Can you work these out from the model? Positions are in its coordinate system, mm. Round coordinates to 2 decimals unless told otherwise and drop trailing zeros. Order: outer loops, then holes, each group sorted by start corner. A loop starts at its lowest first (then second) coordinate and runs counter-clockwise, first axis right, second up. Notation, with made-up numbers: M 63,4.25 L 95,4.25 A23 cw 95,28.25 Z; hole C -4.5,44 d3. An arc over 180 degrees is marked long. Answer as CSV lines item,"result". Start each with the question number.
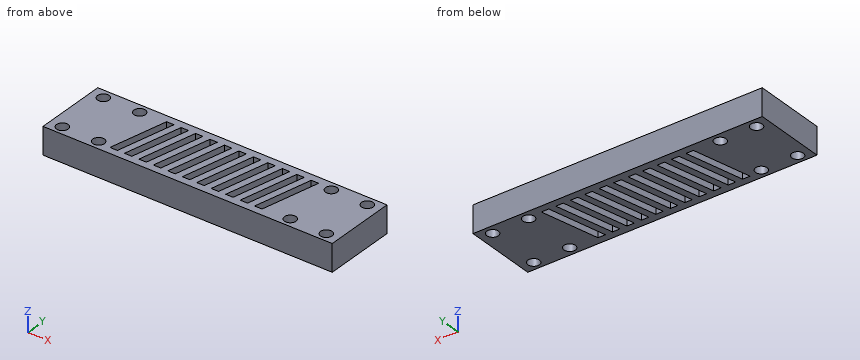
from build123d import *

# Parameters (mm, degrees)
SKETCH1_W           = 80
SKETCH1_H           = 20
SKETCH1_R           = 1.6
BOSS_EXTRUDE4_DEPTH = 7.5
CUT_EXTRUDE1_DEPTH  = 7.5


with BuildPart() as part:
    # Sketch1 → Boss-Extrude4 (new body)
    with BuildSketch(Plane.XY):
        with Locations((0, -0.350941688)):
            Rectangle(SKETCH1_W, SKETCH1_H)
        with Locations((36.5, 7.096795016)):
            Circle(SKETCH1_R, mode=Mode.SUBTRACT)
        with Locations((26.5, 7.149058312)):
            Circle(SKETCH1_R, mode=Mode.SUBTRACT)
        with Locations((36.5, -7.903204984)):
            Circle(SKETCH1_R, mode=Mode.SUBTRACT)
        with Locations((26.5, -7.850941688)):
            Circle(SKETCH1_R, mode=Mode.SUBTRACT)
        with Locations(Location((-26.5, -7.850941688, 0), (0, 0, 180))):  # turned: the seam where the file's is
            Circle(SKETCH1_R, mode=Mode.SUBTRACT)
        with Locations(Location((-36.5, -7.903204984, 0), (0, 0, 180))):  # turned: the seam where the file's is
            Circle(SKETCH1_R, mode=Mode.SUBTRACT)
        with Locations(Location((-26.5, 7.149058312, 0), (0, 0, 180))):  # turned: the seam where the file's is
            Circle(SKETCH1_R, mode=Mode.SUBTRACT)
        with Locations(Location((-36.5, 7.096795016, 0), (0, 0, 180))):  # turned: the seam where the file's is
            Circle(SKETCH1_R, mode=Mode.SUBTRACT)
    extrude(amount=BOSS_EXTRUDE4_DEPTH)

    # Sketch6 → Cut-Extrude1 (cut)
    with BuildSketch(Plane.XY.offset(7.5)):
        Polygon((-19.441029478, 7.649058312), (-22.994766049, -8.350941688), (-20.946027704, -8.350941688), (-17.392291133, 7.649058312), align=None)
        Polygon((-13.392291133, 7.649058312), (-15.441029478, 7.649058312), (-18.994766049, -8.350941688), (-16.946027704, -8.350941688), align=None)
        Polygon((-9.392291133, 7.649058312), (-11.441029478, 7.649058312), (-14.994766049, -8.350941688), (-12.946027704, -8.350941688), align=None)
        Polygon((-5.392291133, 7.649058312), (-7.441029478, 7.649058312), (-10.994766049, -8.350941688), (-8.946027704, -8.350941688), align=None)
        Polygon((-1.392291133, 7.649058312), (-3.441029478, 7.649058312), (-6.994766049, -8.350941688), (-4.946027704, -8.350941688), align=None)
        Polygon((2.607708867, 7.649058312), (0.558970522, 7.649058312), (-2.994766049, -8.350941688), (-0.946027704, -8.350941688), align=None)
        Polygon((6.607708867, 7.649058312), (4.558970522, 7.649058312), (1.005233951, -8.350941688), (3.053972296, -8.350941688), align=None)
        Polygon((10.607708867, 7.649058312), (8.558970522, 7.649058312), (5.005233951, -8.350941688), (7.053972296, -8.350941688), align=None)
        Polygon((14.607708867, 7.649058312), (12.558970522, 7.649058312), (9.005233951, -8.350941688), (11.053972296, -8.350941688), align=None)
        Polygon((18.607708867, 7.649058312), (16.558970522, 7.649058312), (13.005233951, -8.350941688), (15.053972296, -8.350941688), align=None)
        Polygon((22.607708867, 7.649058312), (20.558970522, 7.649058312), (17.005233951, -8.350941688), (19.053972296, -8.350941688), align=None)
    extrude(amount=-CUT_EXTRUDE1_DEPTH, mode=Mode.SUBTRACT)


solid = part.part
(1) I'm going to push a flat-ended pin straight in: P1, Ø3, axis at x = -26.5, y = -7.85, coming from the -Z side. Where does the tip first touch, or does it pass through?
(2) If I drill on line 1 along X through (y, z) = (7.75, 2.75); line 2 along Y through (x, z) = (-37, 5.5); line 3 along Y through (x, z) = (26.5, 3), over which ranges is the centre line in solid material (lowest first)?
(3) I want a section at B-B on z = 4.75. Count the separate pieces of the cut face and the enclosed holes in it, and give its area (3 significant figures).
(4) I want a section at A-A on x = 26.5. Write out the boundary of the cut face in (y, z), and give its area (3 significant figures).
From the geometry:
1,P1,"through"
2,line 1,"-40 to -37.96, -35.04 to -27.98, -25.02 to 25.02, 27.98 to 35.04, 37.96 to 40"
2,line 2,"-10.35 to -9.42, -6.38 to 5.58, 8.62 to 9.65"
2,line 3,"-10.35 to -9.45, -6.25 to 5.55, 8.75 to 9.65"
3,separate pieces,"1"
3,enclosed holes,"19"
3,area,"1,180 mm²"
4,outline,"M -10.35,0 L -9.45,0 L -9.45,7.5 L -10.35,7.5 Z; M -6.25,0 L 5.55,0 L 5.55,7.5 L -6.25,7.5 Z; M 8.75,0 L 9.65,0 L 9.65,7.5 L 8.75,7.5 Z"
4,area,"102 mm²"
